```python
from build123d import *

# Parameters (mm, degrees)
SKETCH_1_R      = 7
EXTRUDE_1_DEPTH = 45
EXTRUDE_2_DEPTH = 7
SKETCH_7_R      = 4
EXTRUDE_3_DEPTH = 135
EXTRUDE_4_DEPTH = 3


with BuildPart() as part:
    # 草图1 → 凸台-拉伸1 (new body)
    with BuildSketch(Plane.XY):
        with Locations(Location((-86.606649797, -63.783530386, 0), (0, 0, 180))):
            Circle(SKETCH_1_R)
    extrude(amount=EXTRUDE_1_DEPTH)

    # 草图3 → 凸台-拉伸2 (add)
    with BuildSketch(Plane(origin=(0, 0, 0), x_dir=(-1, 0, 0), z_dir=(0, 0, -1))):
        with BuildLine():
            Line((87.955581339, -67.549215409), (12.641880873, -94.52784625))
            ThreePointArc((12.641880873, -94.52784625), (7.527264308, -92.111092769), (9.944017789, -86.996476204))
            Line((9.944017789, -86.996476204), (85.257718255, -60.017845362))
            ThreePointArc((85.257718255, -60.017845362), (90.37233482, -62.434598843), (87.955581339, -67.549215409))
        make_face()
    extrude(amount=-EXTRUDE_2_DEPTH)

    # 草图7 → 凸台-拉伸3 (add)
    with BuildSketch(Plane.XY.offset(7)):
        with Locations(Location((-11.292949331, -90.762161227, 0), (0, 0, 250.291624105))):
            Circle(SKETCH_7_R)
    extrude(amount=EXTRUDE_3_DEPTH)

    # 草图8 → 凸台-拉伸4 (add)
    with BuildSketch(Plane.XY.offset(142)):
        Polygon((-15.394140478, -84.335981352), (7.207577452, -92.593097239), (4.030932181, -101.288341605), (-18.57078575, -93.031225719), align=None)
    extrude(amount=EXTRUDE_4_DEPTH)


solid = part.part
```
CAD build for the part. Positions are in the model's coordinates, mm. A direction names the side the tool comes from. Coordinates: 2 decimals unless noted, no trailing zeros. Write each loop counter-clockwise with the first axis right and the second up, starting at its lowest first coordinate (ties: lowest second). Pieces come first, ordered by that corner, then holes. Notation, with made-up numbers: (-15.5, -17) -> (6.5, -17) arc R28 ccw to (6.5, 18) -> close; hole circle Ø10 at (-15, -37.75). An arc over 180 degrees is marked (long way). Return JSON: item names as keys, results as strings. Group by question number.
Q1. Which spindle directions (+Z, -Z, +X, -X, +Y, -Y) get a long thin tool onto all of the face, cutting with end or side? Do faces 1 (the face through (-4.251, -88.407, 143.479)), 2 (the face through (-17.005, -88.744, 143.479)), 3 (the face through (-93.07, -61.1, 22.18)). Say none if no direction does.
Q2. Flat gauge pins, fed straight in: pin 1 (4 mm diameter, centred on x = -9.5, z = 83.5, fed in from +Y); pin 2 (1 mm diameter, centred on x = -14.5, z = 74, fed in from -Y); pin 3 (1 mm diameter, centred on y = -87.5, z = 55.5, fed in from +X). Where does each tip first touch, or does it go through?
Q3. Cut at B-B, the plane z = 81.5. Give the cut face in (x, y), then the cut area to 3 significant figures.
Q4. Cut at C-C, the plane x = -28.5. Give the cut face in (y, z), then the cut area to 3 significant figures.
Q5. Cut at D-D, the plane z = 32.5. Give the cut face in (x, y).
Q6. Drill centre lines: line 1 (X direction, y = -91, z = 10); line 2 (Z direction, x = -3.5, y = -96); line 3 (Z direction, x = -24.5, y = -90). Where is each one in solid material? Low to high.
Q7. Cut at A-A, the plane y = -89. Give the cut face in (x, z), then the cut area to 3 significant figures.
Returned:
{
 "1": {"face 1": "+Z, -Z, +X, +Y", "face 2": "+Z, -X, +Y", "face 3": "+Z"},
 "2": {"pin 1": "stops at y = -86.76", "pin 2": "stops at y = -93.71", "pin 3": "stops at x = -8.4"},
 "3": {"outline": "circle Ø8 at (-11.29, -90.76)", "area": "50.3 mm2"},
 "4": {"outline": "(-88.85, 0) -> (-80.35, 0) -> (-80.35, 7) -> (-88.85, 7) -> close", "area": "59.5 mm2"},
 "5": {"outline": "circle Ø14 at (-86.61, -63.78); circle Ø8 at (-11.29, -90.76)"},
 "6": {"line 1": "x = -15.29 to -7.3", "line 2": "z = 142 to 145", "line 3": "z = 0 to 7"},
 "7": {"outline": "(-28.07, 0) -> (-7.7, 0) -> (-7.7, 142) -> (-2.63, 142) -> (-2.63, 145) -> (-17.1, 145) -> (-17.1, 142) -> (-14.88, 142) -> (-14.88, 7) -> (-28.07, 7) -> close", "area": "1,160 mm2"}
}
